Work out the finished part from the listing and answer in its coordinate system (mm). Round coordinates to 2 decimals unless told otherwise and drop trailing zeros. Write each loop counter-clockwise with the first axis right and the second up, starting at its lowest first coordinate (ties: lowest second). Pieces come first, ordered by that corner, then holes. Notation, with made-up numbers: (-26.5, 4.5) - (-16.5, 4.5) arc R20 cw to (-16.5, 36.5) - close; hole circle Ø10 at (-29.75, 62.5). An arc over 180 degrees is marked (long way). Write item = value, one per line. Start each with the question number.
from build123d import *

# Parameters (mm, degrees)
BOSS_EXTRUDE1_DEPTH = 18.25625
SKETCH2_R           = 1.5875
CUT_EXTRUDE1_DEPTH  = 19.25625
SKETCH3_R           = 1.5875
CUT_EXTRUDE2_DEPTH  = 19.25625


with BuildPart() as part:
    # Sketch1 → Boss-Extrude1 (new body)
    with BuildSketch(Plane.XY):
        with BuildLine():
            Line((0, 990.6), (0, 0))
            Line((0, 0), (457.201, 0))
            Line((457.201, 0), (457.201, 13.862038208))
            ThreePointArc((457.201, 13.862038208), (232.767577124, 176.628269142), (124.367415652, 431.8))
            Line((124.367415652, 431.8), (50.8, 990.6))
            Line((50.8, 990.6), (0, 990.6))
        make_face()
    extrude(amount=BOSS_EXTRUDE1_DEPTH)

    # Sketch2 → Cut-Extrude1 (cut, through all)
    with BuildSketch(Plane.XY.offset(18.25625)):
        with Locations((12.7, 977.9)):
            Circle(SKETCH2_R)
        with Locations((38.1, 977.9)):
            Circle(SKETCH2_R)
        with Locations((12.7, 901.7)):
            Circle(SKETCH2_R)
        with Locations((38.1, 901.7)):
            Circle(SKETCH2_R)
        with Locations((12.7, 609.6)):
            Circle(SKETCH2_R)
        with Locations((38.1, 609.6)):
            Circle(SKETCH2_R)
        with Locations((12.7, 685.8)):
            Circle(SKETCH2_R)
        with Locations((38.1, 685.8)):
            Circle(SKETCH2_R)
        with Locations((12.7, 254)):
            Circle(SKETCH2_R)
        with Locations((38.1, 254)):
            Circle(SKETCH2_R)
        with Locations((12.7, 330.2)):
            Circle(SKETCH2_R)
        with Locations((38.1, 330.2)):
            Circle(SKETCH2_R)
        with Locations((12.7, 38.1)):
            Circle(SKETCH2_R)
        with Locations((12.7, 12.7)):
            Circle(SKETCH2_R)
        with Locations((88.9, 38.1)):
            Circle(SKETCH2_R)
        with Locations((88.9, 12.7)):
            Circle(SKETCH2_R)
        with Locations((241.3, 38.1)):
            Circle(SKETCH2_R)
        with Locations((317.5, 38.1)):
            Circle(SKETCH2_R)
        with Locations((241.3, 12.7)):
            Circle(SKETCH2_R)
        with Locations((317.5, 12.7)):
            Circle(SKETCH2_R)
    extrude(amount=-CUT_EXTRUDE1_DEPTH, mode=Mode.SUBTRACT)

    # Sketch3 → Cut-Extrude2 (cut, through all)
    with BuildSketch(Plane.XY.offset(18.25625)):
        with Locations((88.9, 147.112433493)):
            Circle(SKETCH3_R)
        with Locations((71.4248, 165.527433493)):
            Circle(SKETCH3_R)
        with Locations((155.8036, 165.527433493)):
            Circle(SKETCH3_R)
        with Locations((173.2788, 147.112433493)):
            Circle(SKETCH3_R)
    extrude(amount=-CUT_EXTRUDE2_DEPTH, mode=Mode.SUBTRACT)


solid = part.part
1. Find section C-C on x = 257.5. Give the vertices of the cut face in (y, z), plus the area to 3 significant figures.
2. Find section B-B on y = 872.5. Give the vertices of the cut face in (x, z), plus the area to 3 significant figures.
3. Each of these flat-tipped pins is pushed along its axis until it touches: pin 1 (2 mm diameter, centred on x = 271.5, z = 12.5, fed in from +Y); pin 2 (2.5 mm diameter, centred on x = 38.1, y = 977.9, fed in from +Z); pin 3 (1 mm diameter, centred on y = 189.5, z = 12, fed in from +X); pin 4 (5 mm diameter, centred on y = 793.5, z = 14, fed in from +X). Where does it stop, or does it pass through?
4. Find section A-A on z = 12.75. Give the number of separate pieces and of enclosed holes in the cut face, plus the area to 3 significant figures.
5. Consider line 1 (X direction, y = 609.6, z = 9); line 2 (X direction, y = 977.9, z = 6.5); line 3 (Y direction, x = 317.5, z = 7.5). Determine where each line is inside the solid, lowest interval first.
Answer key:
q1.outline = (0, 0) - (147.81, 0) - (147.81, 18.26) - (0, 18.26) - close
q1.area = 2,700 mm²
q2.outline = (0, 0) - (66.35, 0) - (66.35, 18.26) - (0, 18.26) - close
q2.area = 1,210 mm²
q3.pin_1 = 134.24
q3.pin_2 = through
q3.pin_3 = 223.22
q3.pin_4 = 77.08
q4.separate_pieces = 1
q4.enclosed_holes = 24
q4.area = 150,000 mm²
q5.line_1 = 0 to 11.11, 14.29 to 36.51, 39.69 to 100.96
q5.line_2 = 0 to 11.11, 14.29 to 36.51, 39.69 to 52.47
q5.line_3 = 0 to 11.11, 14.29 to 36.51, 39.69 to 92.35
